Work out the finished part from the listing and answer in its coordinate system (mm). Face numbers are marked on the shaded views. Coordinates: 2 decimals unless noted, no trailing zeros. Loops run counter-clockwise (first coordinate to the right, second up) from the corner with the lowest first, then second, coordinate; pieces in that order, holes last. Notation, with made-up numbers: (43, 29.5) -> (58, 29.5) arc R14 ccw to (58, 48.5) -> close; hole circle Ø1 at (-3, 87.5). An arc over 180 degrees is marked (long way). Use a Markdown table: item, result.
from build123d import *

# Parameters (mm, degrees)
CUT_EXTRUDE_1_REACH      = 101.499
SKETCH_3_R               = 1.6
EXTRUDE_1_DEPTH          = 2
PATTERN_CIRCULAR_1_COUNT = 4


with BuildPart() as part:
    # Sketch 2 → Revolve 1 (revolve)
    with BuildSketch(Plane.XY):
        with BuildLine():
            Line((5, 51.339745962), (25.980762114, 15))
            ThreePointArc((25.980762114, 15), (25.980762114, -15), (0, -30))
            Line((0, -30), (0, -26.5))
            ThreePointArc((0, -26.5), (22.9496732, -13.25), (22.9496732, 13.25))
            Line((22.9496732, 13.25), (1.968911087, 49.589745962))
            Line((1.968911087, 49.589745962), (1.5, 50.401923789))
            Line((1.5, 50.401923789), (1.5, 60))
            Line((1.5, 60), (11, 60))
            Line((11, 60), (11, 56.5))
            Line((11, 56.5), (5, 56.5))
            Line((5, 56.5), (5, 51.339745962))
        make_face()
    revolve(axis=Axis((0, -26.5, 0), (0, -1, 0)))

    # Sketch 3 → Cut-Extrude 1 (cut, up to next)
    with BuildSketch(Plane(origin=(0, 60, 0), x_dir=(1, 0, 0), z_dir=(0, 1, 0)), mode=Mode.PRIVATE) as cut_extrude_1_sk1:
        with Locations(Location((-5.656854249, 5.656854249, 0), (0, 0, 180))):
            Circle(SKETCH_3_R)
    cut_extrude_1_tool1 = extrude(cut_extrude_1_sk1.sketch, amount=-CUT_EXTRUDE_1_REACH, mode=Mode.PRIVATE) & part.part
    # Sketch 3 → Cut-Extrude 1 (cut, up to next)
    with BuildSketch(Plane(origin=(0, 60, 0), x_dir=(1, 0, 0), z_dir=(0, 1, 0)), mode=Mode.PRIVATE) as cut_extrude_1_sk2:
        with Locations(Location((5.656854249, 5.656854249, 0), (0, 0, 180))):
            Circle(SKETCH_3_R)
    cut_extrude_1_tool2 = extrude(cut_extrude_1_sk2.sketch, amount=-CUT_EXTRUDE_1_REACH, mode=Mode.PRIVATE) & part.part
    # Sketch 3 → Cut-Extrude 1 (cut, up to next)
    with BuildSketch(Plane(origin=(0, 60, 0), x_dir=(1, 0, 0), z_dir=(0, 1, 0)), mode=Mode.PRIVATE) as cut_extrude_1_sk3:
        with Locations(Location((5.656854249, -5.656854249, 0), (0, 0, 180))):
            Circle(SKETCH_3_R)
    cut_extrude_1_tool3 = extrude(cut_extrude_1_sk3.sketch, amount=-CUT_EXTRUDE_1_REACH, mode=Mode.PRIVATE) & part.part
    # Sketch 3 → Cut-Extrude 1 (cut, up to next)
    with BuildSketch(Plane(origin=(0, 60, 0), x_dir=(1, 0, 0), z_dir=(0, 1, 0)), mode=Mode.PRIVATE) as cut_extrude_1_sk4:
        with Locations(Location((-5.656854249, -5.656854249, 0), (0, 0, 180))):
            Circle(SKETCH_3_R)
    cut_extrude_1_tool4 = extrude(cut_extrude_1_sk4.sketch, amount=-CUT_EXTRUDE_1_REACH, mode=Mode.PRIVATE) & part.part
    add(cut_extrude_1_tool1.solids().sort_by_distance((-5.656854, 60, -5.656854))[0], mode=Mode.SUBTRACT)
    add(cut_extrude_1_tool2.solids().sort_by_distance((5.656854, 60, -5.656854))[0], mode=Mode.SUBTRACT)
    add(cut_extrude_1_tool3.solids().sort_by_distance((5.656854, 60, 5.656854))[0], mode=Mode.SUBTRACT)
    add(cut_extrude_1_tool4.solids().sort_by_distance((-5.656854, 60, 5.656854))[0], mode=Mode.SUBTRACT)

    # Sketch 4 → Extrude 1 (add, symmetric)
    with BuildSketch(Plane.XY):
        Polygon((-5, 51.339745962), (-7.979274058, 56.5), (-8.520148677, 57.436822322), (-4.121868793, 57.436822322), (-4.121868793, 49.818778096), align=None)
    extrude_1 = extrude(amount=EXTRUDE_1_DEPTH, both=True)

    # Pattern Circular 1: Extrude 1 ×4 about axis
    pattern_circular_1_axis = Axis((0, 0, 0), (0, 1, 0))
    for i in range(1, PATTERN_CIRCULAR_1_COUNT):
        add(extrude_1.rotate(pattern_circular_1_axis, i * 360 / PATTERN_CIRCULAR_1_COUNT))


solid = part.part
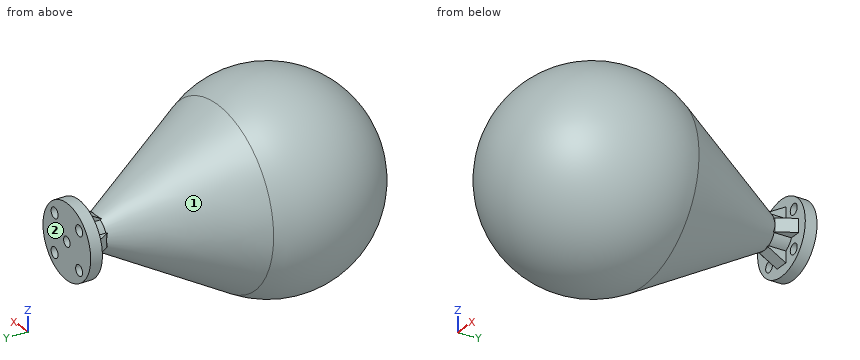
Q1. Determine the mould class of the marked faces 1 and 2 for opening direction Y: pulls with the +Y half, pulls with the -Y half, needs draft (parallel to the pull), parting line crosses it, or undercut.
Solved:
| item | result |
|---|---|
| face 1 | undercut |
| face 2 | pulls with the +Y half |
Q2. Consider line 1 (Y direction, x = -1.5, z = -10); line 2 (X direction, y = 17, z = 5.5); line 3 (X direction, y = -4, z = -6). Determine where each line is inside the solid, lowest interval first. Write a range as [from, to].
Solved:
| item | result |
|---|---|
| line 1 | [-28.24, -24.49], [35.49, 42.49], [56.5, 60] |
| line 2 | [-24.21, -20.04], [20.04, 24.21] |
| line 3 | [-29.12, -25.5], [25.5, 29.12] |
Q3. Section A-A on x = 6 is taken. State how many separate pieces and enclosed holes the cut face has, and give its area (3 significant figures).
Solved:
| item | result |
|---|---|
| separate pieces | 4 |
| enclosed holes | 1 |
| area | 805 mm² |
Q4. Given pin 1 Ø4 at (x, z) = (-22, 8.5) entering from -Y; pin 2 Ø3.5 at (x, y) = (7, 54.5) entering from +Z; pin 3 Ø1 at (y, z) = (14.5, 2.5) entering from -X; pin 4 Ø4 at (x, z) = (5.66, 5.66) entering from +Y, each flat-ended and moving along its own axis, determine where each tip first touches the part or whether it passes through.
Solved:
| item | result |
|---|---|
| pin 1 | y = -20.83 |
| pin 2 | z = 2 |
| pin 3 | x = -26.42 |
| pin 4 | y = 60 |
Q5. Section C-C on y = 35 is taken. Determine the outline of the cut face in (x, z), and give its area (3 significant figures).
Solved:
| item | result |
|---|---|
| outline | circle Ø28.87 at (0, 0); hole circle Ø20.78 at (0, 0) |
| area | 315 mm² |
Q6. Section B-B on y = 25 is taken. Determine the outline of the cut face in (x, z), and give its area (3 significant figures).
Solved:
| item | result |
|---|---|
| outline | circle Ø40.41 at (0, 0); hole circle Ø32.33 at (0, 0) |
| area | 462 mm² |
